Geometry check sheet. Reference: the model listing, model coordinates, mm. Give positions to 0.01 mm unless a question says otherwise; leave off trailing zeros. Loops run counter-clockwise (first coordinate to the right, second up) from the corner with the lowest first, then second, coordinate; pieces in that order, holes last. Notation, with made-up numbers: (62.25, 11.5) -> (94.25, 11.5) arc R12 cw to (94.25, 23.5) -> close; hole circle Ø2 at (81.25, 86). An arc over 180 degrees is marked (long way). Write each question's results on one line, items separated by ' | '. Start each with the question number.
1) Sectioned sample at C-C on z = 20.5. Record the cut outline in (x, y).
2) Draft check along X on faces 1 (the face through (0.15, 9.14, 21.41)), 2 (the face through (-13.986, 0.616, 19.72)), 3 (the face through (-0.867, -3.905, 19.72)). Enter one of: pulls with the +X half, pulls with the -X half, needs draft (parallel to the pull), parting line crosses it, or undercut.
3) Sectioned sample at D-D on x = -7.25. Record the cut outline in (y, z), then the cut area to 3 significant figures.
4) Sectioned sample at B-B on x = 0. Record the cut outline in (y, z), then the cut area to 3 significant figures.
5) Sectioned sample at A-A on y = 0. Record the cut outline in (x, z).
6) Scan lines: line 1 (X direction, y = 1.5, z = 35); line 2 (X direction, y = -3, z = 7); line 3 (Z direction, x = 6.5, y = 9.5). Record each from-to range of solid material in increasing order. Write a range as from..to.
7) Depth check by flat-ended pin: pin 1 (5 mm diameter, centred on x = 11, z = 13.5, fed in from +Y); pin 2 (2 mm diameter, centred on y = 10, z = 6.5, fed in from +X); pin 3 (5 mm diameter, centred on y = 1.5, z = 14, fed in from -X); pin 4 (7 mm diameter, centred on y = 12.14, z = 11.31, fed in from +X). Enter the tip coordinate at first touch or a pass-through.
```python
from build123d import *

# Parameters (mm, degrees)
SKETCH1_R               = 14
SKETCH1_R_2             = 4
EXTRUDE_THIN1_DEPTH     = 40
SKETCH2_R               = 3
CUT_EXTRUDE1_DEPTH      = 15
CUT_EXTRUDE1_DEPTH_BACK = 15


with BuildPart() as part:
    # Sketch1 → Extrude-Thin1 (new body)
    with BuildSketch(Plane.XY):
        Circle(SKETCH1_R)
        Circle(SKETCH1_R_2, mode=Mode.SUBTRACT)
    extrude(amount=EXTRUDE_THIN1_DEPTH)

    # Sketch2 → Cut-Extrude1 (cut, two sides)
    with BuildSketch(Plane(origin=(0, 0, 0), x_dir=(0, 0, -1), z_dir=(1, 0, 0))) as cut_extrude1_sk:
        with Locations((-31.312329447, 12.13670973)):
            Circle(SKETCH2_R)
        with Locations((-21.312329447, 12.13670973)):
            Circle(SKETCH2_R)
        with Locations((-11.312329447, 12.13670973)):
            Circle(SKETCH2_R)
        with Locations((-21.312329447, -12.86329027)):
            Circle(SKETCH2_R)
        with Locations((-11.312329447, -12.86329027)):
            Circle(SKETCH2_R)
        with Locations((-31.312329447, -12.86329027)):
            Circle(SKETCH2_R)
    extrude(amount=CUT_EXTRUDE1_DEPTH, mode=Mode.SUBTRACT)
    extrude(cut_extrude1_sk.sketch, amount=-CUT_EXTRUDE1_DEPTH_BACK, mode=Mode.SUBTRACT)


solid = part.part
```
Result:
1) outline: (-10.51, 9.25) arc R14 ccw to (-9.82, -9.98) -> (9.82, -9.98) arc R14 ccw to (10.51, 9.25) -> close; hole circle Ø8 at (0, 0)
2) face 1: needs draft | face 2: parting line crosses it | face 3: undercut
3) outline: (-11.98, 0) -> (11.98, 0) -> (11.98, 8.32) arc R3 cw to (11.98, 14.31) -> (11.98, 18.32) arc R3 cw to (11.98, 24.31) -> (11.98, 28.32) arc R3 cw to (11.98, 34.31) -> (11.98, 40) -> (-11.98, 40) -> (-11.98, 34.18) arc R3 cw to (-11.98, 28.45) -> (-11.98, 24.18) arc R3 cw to (-11.98, 18.45) -> (-11.98, 14.18) arc R3 cw to (-11.98, 8.45) -> close | area: 892 mm^2
4) outline: (-14, 0) -> (-4, 0) -> (-4, 40) -> (-14, 40) -> (-14, 34.09) arc R3 cw (long way) to (-14, 28.54) -> (-14, 24.09) arc R3 cw (long way) to (-14, 18.54) -> (-14, 14.09) arc R3 cw (long way) to (-14, 8.54) -> close; (4, 0) -> (14, 0) -> (14, 8.96) arc R3 cw (long way) to (14, 13.66) -> (14, 18.96) arc R3 cw (long way) to (14, 23.66) -> (14, 28.96) arc R3 cw (long way) to (14, 33.66) -> (14, 40) -> (4, 40) -> close | area: 664 mm^2
5) outline: (-14, 0) -> (-4, 0) -> (-4, 40) -> (-14, 40) -> close; (4, 0) -> (14, 0) -> (14, 40) -> (4, 40) -> close
6) line 1: -13.92..-3.71, 3.71..13.92 | line 2: -13.67..-2.65, 2.65..13.67 | line 3: 0..9.88, 12.74..19.88, 22.74..29.88, 32.74..40
7) pin 1: y = 11.07 | pin 2: x = 10.72 | pin 3: x = -14 | pin 4: x = 11.02
